The listing builds one solid part. Answer for the finished solid, in the listing's coordinates (mm). A direction names the side the tool comes from. Coordinates: 2 decimals unless noted, no trailing zeros. Write each loop counter-clockwise with the first axis right and the second up, starting at its lowest first coordinate (ties: lowest second). Pieces come first, ordered by that corner, then holes. Notation, with made-up numbers: M -27.5,-18 L 4.5,-18 A30 cw 4.5,10 Z; hole C 60,3 d7. An arc over 180 degrees is marked long. Answer as CSV lines item,"result".
```python
from build123d import *

# Parameters (mm, degrees)
SKETCH_1_W          = 97.7
SKETCH_1_H          = 148.7
EXTRUDE_1_DEPTH     = 3
FILLET_1_R          = 5
CUT_EXTRUDE_1_REACH = 91.013
SKETCH_2_R          = 1.6
SKETCH_3_R          = 15
EXTRUDE_2_DEPTH     = 3
CUT_EXTRUDE_2_DEPTH = 4.5
CUT_EXTRUDE_START   = 3
SKETCH_5_R          = 12.5
CUT_EXTRUDE_3_DEPTH = 3
SKETCH_6_W          = 10.2
SKETCH_6_H          = 120.3
SKETCH_6_W_2        = 30.1
SKETCH_6_H_2        = 10.1
CUT_EXTRUDE_4_DEPTH = 2.1


with BuildPart() as part:
    # 草图1 → 凸台-拉伸1 (new body)
    with BuildSketch(Plane.XY):
        Rectangle(SKETCH_1_W, SKETCH_1_H)
    extrude(amount=EXTRUDE_1_DEPTH)

    # 圆角1
    fillet_1_edges = [part.edges().sort_by_distance(p)[0] for p in [
        (-48.85, 74.35, 1.5),
        (48.85, 74.35, 1.5),
        (48.85, -74.35, 1.5),
        (-48.85, -74.35, 1.5),
    ]]
    fillet(fillet_1_edges, radius=FILLET_1_R)

    # 草图2 → 切除-拉伸1 (cut, up to next)
    with BuildSketch(Plane.XY.offset(3), mode=Mode.PRIVATE) as cut_extrude_1_sk1:
        with Locations((-44, 69.5)):
            Circle(SKETCH_2_R)
    cut_extrude_1_tool1 = extrude(cut_extrude_1_sk1.sketch, amount=-CUT_EXTRUDE_1_REACH, mode=Mode.PRIVATE) & part.part
    # 草图2 → 切除-拉伸1 (cut, up to next)
    with BuildSketch(Plane.XY.offset(3), mode=Mode.PRIVATE) as cut_extrude_1_sk2:
        with Locations((44, 69.5)):
            Circle(SKETCH_2_R)
    cut_extrude_1_tool2 = extrude(cut_extrude_1_sk2.sketch, amount=-CUT_EXTRUDE_1_REACH, mode=Mode.PRIVATE) & part.part
    # 草图2 → 切除-拉伸1 (cut, up to next)
    with BuildSketch(Plane.XY.offset(3), mode=Mode.PRIVATE) as cut_extrude_1_sk3:
        with Locations((-44, -69.5)):
            Circle(SKETCH_2_R)
    cut_extrude_1_tool3 = extrude(cut_extrude_1_sk3.sketch, amount=-CUT_EXTRUDE_1_REACH, mode=Mode.PRIVATE) & part.part
    # 草图2 → 切除-拉伸1 (cut, up to next)
    with BuildSketch(Plane.XY.offset(3), mode=Mode.PRIVATE) as cut_extrude_1_sk4:
        with Locations((44, -69.5)):
            Circle(SKETCH_2_R)
    cut_extrude_1_tool4 = extrude(cut_extrude_1_sk4.sketch, amount=-CUT_EXTRUDE_1_REACH, mode=Mode.PRIVATE) & part.part
    add(cut_extrude_1_tool1.solids().sort_by_distance((-44, 69.5, 3))[0], mode=Mode.SUBTRACT)
    add(cut_extrude_1_tool2.solids().sort_by_distance((44, 69.5, 3))[0], mode=Mode.SUBTRACT)
    add(cut_extrude_1_tool3.solids().sort_by_distance((-44, -69.5, 3))[0], mode=Mode.SUBTRACT)
    add(cut_extrude_1_tool4.solids().sort_by_distance((44, -69.5, 3))[0], mode=Mode.SUBTRACT)

    # 草图3 → 凸台-拉伸2 (add)
    with BuildSketch(Plane.XY.offset(3)):
        with Locations((0, 34.65)):
            Circle(SKETCH_3_R)
    extrude(amount=EXTRUDE_2_DEPTH)

    # 草图4 → 切除-拉伸2 (cut)
    with BuildSketch(Plane(origin=(0, 0, 0), x_dir=(-1, 0, 0), z_dir=(0, 0, -1))):
        with BuildLine():
            Line((-12.5, 34.65), (12.5, 34.65))
            ThreePointArc((12.5, 34.65), (0, 22.15), (-12.5, 34.65))
        make_face()
    extrude(amount=-CUT_EXTRUDE_2_DEPTH, mode=Mode.SUBTRACT)

    # 草图5 → 切除-拉伸3 (cut)
    with BuildSketch(Plane(origin=(0, 0, 4.5), x_dir=(-1, 0, 0), z_dir=(0, 0, -1)).offset(CUT_EXTRUDE_START)):
        with Locations((0, 34.65)):
            Circle(SKETCH_5_R)
    extrude(amount=-CUT_EXTRUDE_3_DEPTH, mode=Mode.SUBTRACT)

    # 草图6 → 切除-拉伸4 (cut)
    with BuildSketch(Plane(origin=(0, 0, 0), x_dir=(-1, 0, 0), z_dir=(0, 0, -1))):
        with Locations((-33.75, -4.2)):
            Rectangle(SKETCH_6_W, SKETCH_6_H)
        Polygon((28.65, 55.9), (32.118068627, -64.35), (38.85, -64.35), (38.85, 55.9), align=None)
        with Locations((0, 61)):
            Rectangle(SKETCH_6_W_2, SKETCH_6_H_2)
        with Locations((0, -59.3)):
            Rectangle(SKETCH_6_W_2, SKETCH_6_H_2)
    extrude(amount=-CUT_EXTRUDE_4_DEPTH, mode=Mode.SUBTRACT)


solid = part.part
```
Q1. Find section D-D (y = 7). Give the vertices of the cut face in (x, z), and give its area (3 significant figures).
Output:
outline,"M -48.85,0 L -38.85,0 L -38.85,2.1 L -30.06,2.1 L -30.06,0 L 28.65,0 L 28.65,2.1 L 38.85,2.1 L 38.85,0 L 48.85,0 L 48.85,3 L -48.85,3 Z"
area,"253 mm2"
Q2. Find section C-C (x = 35). Give the vertices of the cut face in (y, z), and give its area (3 significant figures).
Output:
outline,"M -74.35,0 L -64.35,0 L -64.35,2.1 L 55.95,2.1 L 55.95,0 L 74.35,0 L 74.35,3 L -74.35,3 Z"
area,"193 mm2"
Q3. For faces 1 (the cylindrical face through (1.627, 22.256, 2.718)), 2 (the flat face through (0, 61, 2.1)), 3 (the cylindrical face through (-44.208, -67.914, 1.521)), determine the directions among +Z, -Z, +X, -X, +Y, -Y from which every point of the face is accessible in a straight line to the end or side of a thin tool.
Output:
face 1,"none"
face 2,"-Z"
face 3,"+Z, -Z"
Q4. Flat-ended cylindrical pins translate along their axes: pin 1 Ø2 at (x, z) = (-9, 5) entering from -Y; pin 2 Ø1.9 at (x, y) = (44, 69.5) entering from +Z; pin 3 Ø5 at (x, y) = (7, 63) entering from -Z. Find the tip coordinate at first contact, or state that the pin passes through.
Output:
pin 1,"y = 21.96"
pin 2,"through"
pin 3,"z = 2.1"
Q5. Find section B-B (y = -33). Give the vertices of the cut face in (x, z).
Output:
outline,"M -48.85,0 L -38.85,0 L -38.85,2.1 L -31.21,2.1 L -31.21,0 L 28.65,0 L 28.65,2.1 L 38.85,2.1 L 38.85,0 L 48.85,0 L 48.85,3 L -48.85,3 Z"
Q6. Straight lines are drawn through the part: line 1 (X direction, y = -69.5, z = 2.4); line 2 (Y direction, x = -44, z = 1.4); line 3 (Y direction, x = 9, z = 0.35). For each, find the intervals that lie inside material, in ascending order.
Output:
line 1,"-48.85 to -45.6, -42.4 to 42.4, 45.6 to 48.85"
line 2,"-74.35 to -71.1, -67.9 to 67.9, 71.1 to 74.35"
line 3,"-74.35 to -64.35, -54.25 to 25.98, 34.65 to 55.95, 66.05 to 74.35"
Q7. The mould has two halves that part along Y. Classify faces 4 (the flat face through (-1, -74.35, 1)), 5 (the cylindrical face through (-3.252, 20.007, 4.479)), 6 (the flat face through (0, 35, 4.5)): pulls with the +Y half, pulls with the -Y half, needs draft (parallel to the pull), parting line crosses it, or undercut.
Output:
face 4,"pulls with the -Y half"
face 5,"parting line crosses it"
face 6,"undercut"
Q8. Find section A-A (x = -36.5). Give the vertices of the cut face in (y, z).
Output:
outline,"M -74.35,0 L -64.35,0 L -64.35,2.1 L 55.9,2.1 L 55.9,0 L 74.35,0 L 74.35,3 L -74.35,3 Z"
